Input: part model. Units: mm. Frame: model coordinates. A direction names the side the tool comes from. Round coordinates to 2 decimals unless told otherwise and drop trailing zeros. Order: outer loops, then holes, each group sorted by start corner. A loop starts at its lowest first (then second) coordinate and runs counter-clockwise, first axis right, second up. Notation, with made-up numbers: M 29.25,66 L 67.25,66 A21 ccw 67.25,74 Z; hole C -24,-11.5 d3. An arc over 180 degrees is marked long. One line per question, with ' | ' between items.
Autodesk Inventor part; units mm, degrees
ref_plane "YZ Plane" through (0, 0, 0) normal (1, 0, 0) x (0, 1, 0)
ref_plane "XZ Plane" through (0, 0, 0) normal (0, 1, 0) x (-1, 0, 0)
ref_plane "XY Plane" through (0, 0, 0) normal (0, 0, 1) x (1, 0, 0)
sketch "Эскиз1" plane through (0, 0, 0) normal (0, 1, 0) x (-1, 0, 0)
  line L0 (0, 14.2) -> (24.4, 14.2)
  line L1 (24.4, 14.2) -> (24.4, -14.2)
  line L2 (24.4, -14.2) -> (0, -14.2)
  line L3 (0, -14.2) -> (0, 0)
  line L4 (0, 0) -> (0, 14.2)
  point P0 (24.4, 0)
  dimension "d0" = 24.4
  dimension "d1" = 28.4
extrude "Выдавливание1" add sketch "Эскиз1" along normal blind 4
sketch "Эскиз2" plane through (0, 4, 0) normal (0, 1, 0) x (1, 0, 0)
  line L0 (-23.2, -13) -> (-1.2, -13)
  line L1 (-1.2, -13) -> (-1.2, 13)
  line L2 (-1.2, 13) -> (-23.2, 13)
  line L3 (-23.2, 13) -> (-23.2, -13)
  line L4 (0, 14.2) -> (-24.4, 14.2)
  line L5 (-24.4, 14.2) -> (-24.4, -14.2)
  line L6 (-24.4, -14.2) -> (0, -14.2)
  line L7 (0, -14.2) -> (0, 14.2)
  line L8 (0, 14.2) -> (-24.4, 14.2)
  line L9 (-24.4, 14.2) -> (-24.4, -14.2)
  point P0 (0, 0)
  point P1 (-12.2, 13)
  point P2 (-12.2, 14.2)
  point P3 (-23.2, 0)
  point P4 (-24.4, 0)
  dimension "d4" = 26
  dimension "d5" = 22
extrude "Выдавливание2" add sketch "Эскиз2" along normal blind 1.6
sketch "Эскиз4" plane through (-24.4, 0, 14.2) normal (0, 0, 1) x (1, 0, 0)
  line L0 (6.2, 0) -> (18.2, 0)
  line L1 (18.2, 0) -> (18.2, 3)
  line L2 (18.2, 3) -> (6.2, 3)
  line L3 (6.2, 3) -> (6.2, 0)
  line L4 (0, 0) -> (24.4, 0)
  point P0 (12.2, 0)
  dimension "d8" = 3
  dimension "d9" = 12
extrude "Выдавливание3" add sketch "Эскиз4" along normal blind 8
chamfer "Фаска1" distance 3 angle 45 2 edges at (-6.2, 1.5, 22.2) (-18.2, 1.5, 22.2)
mirror "Зеркальное отражение1" about plane through (0, 0, 0) normal (0, 0, 1) of "Выдавливание3", "Фаска1"
sketch "Эскиз6" plane through (-18.2, 3, 14.2) normal (0, 1, 0) x (1, 0, 0)
  line L0 (9, 36.4) -> (3, 36.4)
  line L1 (-5, 27.2) -> (-5, 1.2)
  line L2 (-5, 14.2) -> (17, 14.2)
  line L3 (17, 1.2) -> (17, 27.2)
  point P0 (18.2, 14.2)
  point P1 (6, -3.8)
  point P2 (6, 32.2)
  point P3 (6, 36.4)
  dimension "d23" = 36
hole "Отверстие1" at (-12.2, 3, 18) at (-12.2, 3, -18) direction (0, -1, 0) diameter 3.2 end through all
sketch "Эскиз7" plane through (0, 4, 0) normal (0, 1, 0) x (1, 0, 0)
  line L0 (-23.2, 13) -> (-1.2, 13)
  line L1 (-23.2, -13) -> (-23.2, 13)
  line L2 (-1.2, 13) -> (-1.2, -13)
  point P0 (0, 0)
  point P1 (-10.2, 9.6)
  dimension "d31" = 3.4
  dimension "d33" = 9
hole "Отверстие2" at (-10.2, 4, -9.6) direction (0, -1, 0) diameter 2.8 end through all
properties part number "driver"
Item 1: Section query A-A, the plane z = -9.6. Return loops of the section in (x, y), plus the area to 3 significant figures.
Report:
outline: M -24.4,0 L -11.6,0 L -11.6,4 L -23.2,4 L -23.2,5.6 L -24.4,5.6 Z; M -8.8,0 L 0,0 L 0,5.6 L -1.2,5.6 L -1.2,4 L -8.8,4 Z | area: 90.2 mm²
Item 2: Access query for faces 1 (the flat face through (-23.2, 5, 0)), 2 (the flat face through (-6.2, 2, -17)), 3 (the flat face through (-12, 3, 16)). Directions: +Z, -Z, +X, -X, +Y, -Y. A direction counts if a zero-diameter tool reaches every point of the face in a straight line with its end or side. Return the directions, or none.
Report:
face 1: +Y | face 2: -Z, +X, +Y, -Y | face 3: +Z, +X, -X, +Y
Item 3: Section query D-D, the plane z = -1.5. Return loops of the section in (x, y), plus the area to 3 significant figures.
Report:
outline: M -24.4,0 L 0,0 L 0,5.6 L -1.2,5.6 L -1.2,4 L -23.2,4 L -23.2,5.6 L -24.4,5.6 Z | area: 101 mm²
Item 4: First-contact query: pin 1 (9 mm diameter, centred on x = -12.5, z = -20, fed in from +Y); pin 2 (3 mm diameter, centred on y = 2, z = -17, fed in from -X); pin 3 (6 mm diameter, centred on x = -20.5, z = 17, fed in from -Y); pin 4 (6.5 mm diameter, centred on x = -17, z = -1.5, fed in from +Y). Flat tips, straight axial feed; report the tip coordinate or a pass-through.
Report:
pin 1: y = 3 | pin 2: x = -18.2 | pin 3: y = 0 | pin 4: y = 4
Item 5: Section query B-B, the plane y = 4.85. Return loops of the section in (x, z), plus the area to 3 significant figures.
Report:
outline: M -24.4,-14.2 L 0,-14.2 L 0,14.2 L -24.4,14.2 Z; hole M -23.2,-13 L -1.2,-13 L -1.2,13 L -23.2,13 Z | area: 121 mm²
Item 6: Section query C-C, the plane x = -12.2. Return loops of the section in (y, z), plus the area to 3 significant figures.
Report:
outline: M 0,-22.2 L 3,-22.2 L 3,-19.6 L 0,-19.6 Z; M 0,-16.4 L 3,-16.4 L 3,-14.2 L 5.6,-14.2 L 5.6,-13 L 4,-13 L 4,13 L 5.6,13 L 5.6,14.2 L 3,14.2 L 3,16.4 L 0,16.4 Z; M 0,19.6 L 3,19.6 L 3,22.2 L 0,22.2 Z | area: 146 mm²
Item 7: Line query: line 1 along Z through (x, y) = (-12.2, 1.3); line 2 along Z through (x, y) = (-10.2, 2.3); line 3 along X through (y, z) = (1.9, -18). Output: solid intervals per line, ascending. Write a range as from..to.
Report:
line 1: -22.2..-19.6, -16.4..16.4, 19.6..22.2 | line 2: -22.2..-11, -8.2..22.2 | line 3: -18.2..-13.8, -10.6..-6.2
Item 8: Mould query, pull axis X, two halves, no side actions, for faces 4 (the flat face through (-18.2, 1, -17)), 5 (the cylindrical face through (-10.64, 1.48, 17.65)), 6 (the flat face through (-6.2, 1, 17)). Classes: +X half, -X half, draft (parallel to the pull), parting line (faces both ways), or undercut.
Report:
face 4: -X half | face 5: undercut | face 6: +X half
